from build123d import *

# Parameters (mm, degrees)
SKETCH_W        = 98
SKETCH_H        = 58
SKETCH_W_2      = 95
SKETCH_H_2      = 55
PAD_DEPTH       = 65
SKETCH001_W     = 98
SKETCH001_H     = 58
PAD001_DEPTH    = 1.5
SKETCH002_R     = 15.5
POCKET_DEPTH    = 5
SKETCH004_R     = 18.25
POCKET002_DEPTH = 0.75
SKETCH003_W     = 14.5
SKETCH003_H     = 12
SKETCH003_W_2   = 13
SKETCH003_H_2   = 6
SKETCH003_W_3   = 8
SKETCH003_H_3   = 4
POCKET003_DEPTH = 5
PAD002_DEPTH    = 3
PAD003_DEPTH    = 1


with BuildPart() as part:
    # Sketch → Pad (new body)
    with BuildSketch(Plane.XY):
        with Locations((0, -29)):
            Rectangle(SKETCH_W, SKETCH_H)
        with Locations((0, -29)):
            Rectangle(SKETCH_W_2, SKETCH_H_2, mode=Mode.SUBTRACT)
    extrude(amount=PAD_DEPTH)

    # Sketch001 → Pad001 (join)
    with BuildSketch(Plane.XY):
        with Locations((0, -29)):
            Rectangle(SKETCH001_W, SKETCH001_H)
    extrude(amount=PAD001_DEPTH)

    # Sketch002 → Pocket (cut)
    with BuildSketch(Plane.XZ):
        with Locations((0, 30)):
            Circle(SKETCH002_R)
    extrude(amount=POCKET_DEPTH, mode=Mode.SUBTRACT)

    # Sketch004 → Pocket002 (cut)
    with BuildSketch(Plane.XZ.offset(1.5)):
        with Locations((0, 30)):
            Circle(SKETCH004_R)
    extrude(amount=-POCKET002_DEPTH, mode=Mode.SUBTRACT)

    # Sketch003 → Pocket003 (cut)
    with BuildSketch(Plane.XY):
        with Locations((0, -8.5)):
            Rectangle(SKETCH003_W, SKETCH003_H)
        with Locations((31, -46)):
            Rectangle(SKETCH003_W_2, SKETCH003_H_2)
        with Locations((16.2, -46)):
            Rectangle(SKETCH003_W_3, SKETCH003_H_3)
    extrude(amount=POCKET003_DEPTH, mode=Mode.SUBTRACT)

    # Sketch005 → Pad002 (join)
    with BuildSketch(Plane.XZ):
        with BuildLine():
            ThreePointArc((23.5, 30), (0, 53.5), (-23.5, 30))
            Line((-25, 30), (-23.5, 30))
            ThreePointArc((25, 30), (0, 55), (-25, 30))
            Line((23.5, 30), (25, 30))
        make_face()
    extrude(amount=-PAD002_DEPTH)

    # Sketch006 (on Face33 of Pad002) → Pad003 (join)
    with BuildSketch(Plane(origin=(0, 3, 0), x_dir=(-1, 0, 0), z_dir=(0, 1, 0))):
        with BuildLine():
            ThreePointArc((26.5, 30), (0, 56.5), (-26.5, 30))
            Line((-26.5, 30), (-23.5, 30))
            ThreePointArc((23.5, 30), (0, 53.5), (-23.5, 30))
            Line((23.5, 30), (26.5, 30))
        make_face()
    extrude(amount=-PAD003_DEPTH)


solid = part.part
Read the model definition and answer for the solid it produces. Units are mm, in the model's axes. A direction names the side the tool comes from. Round coordinates to 2 decimals unless told otherwise and drop trailing zeros. Write each loop counter-clockwise with the first axis right and the second up, starting at its lowest first coordinate (ties: lowest second). Pieces come first, ordered by that corner, then holes. Notation, with made-up numbers: (1, 16.25) - (10, 16.25) arc R26 ccw to (10, 55.25) - close; hole circle Ø8 at (4.5, -7.5). An arc over 180 degrees is marked (long way). One line per question, with ' | ' between items. Start each with the question number.
1. Section B-B (z = 6.5) is taken. Determine the outline of the cut face in (x, y).
2. Section C-C (y = -10) is taken. Determine the outline of the cut face in (x, z), and give its area (3 significant figures).
3. Find the intervals of material crossed by probe 1 along Y at (x, z) = (-23.5, 10); probe 2 along X at (y, z) = (-5.5, 17.5); probe 3 along Y at (x, z) = (-14.5, 24), in increasing order. Write a range as [from, to].
4. Section A-A (x = 0) is taken. Determine the outline of the cut face in (y, z).
5. Section D-D (x = -10) is taken. Determine the outline of the cut face in (y, z).
6. This flat-tipped pin is pushed along its axis until it touches: pin 1 (1.5 mm diameter, centred on x = -35.5, y = -7, fed in from +Z). Where does it stop, or does it pass through?
7. For faces 1 (the face through (24.7, 1.9, 30)), 2 (the face through (-11, -1.5, 47)), 3 (the face through (-3.956, -1.13, 12.184)), 4 (the face through (0.517, 1.479, 53.494)), 5 (the face through (-0.583, 2.507, 56.494)), determine the directions among +Z, -Z, +X, -X, +Y, -Y from which every point of the face is accessible in a straight line to the end or side of a thin tool.
8. For a pull along Z with two mould halves and no side action, classify faces 6 (the face through (0.55, 0.986, 54.994)), 7 (the face through (-8.2, -0.75, 16.6)), 8 (the face through (-24.6, 1.9, 30)) as +Z half, -Z half, draft (parallel to the pull), parting line (faces both ways), or undercut.
Filled in:
1) outline: (-49, -58) - (49, -58) - (49, 0) - (-49, 0) - close; hole (-47.5, -56.5) - (47.5, -56.5) - (47.5, -1.5) - (-47.5, -1.5) - close
2) outline: (-49, 0) - (-7.25, 0) - (-7.25, 1.5) - (-47.5, 1.5) - (-47.5, 65) - (-49, 65) - close; (7.25, 0) - (49, 0) - (49, 65) - (47.5, 65) - (47.5, 1.5) - (7.25, 1.5) - close | area: 316 mm²
3) probe 1: [-58, -56.5], [-1.5, 0] | probe 2: [-49, -47.5], [47.5, 49] | probe 3: [-58, -56.5], [-0.75, 0]
4) outline: (-58, 0) - (-14.5, 0) - (-14.5, 1.5) - (-56.5, 1.5) - (-56.5, 65) - (-58, 65) - close; (-2.5, 0) - (0, 0) - (0, 14.5) - (-0.75, 14.5) - (-0.75, 11.75) - (-1.5, 11.75) - (-1.5, 1.5) - (-2.5, 1.5) - close; (-1.5, 48.25) - (-0.75, 48.25) - (-0.75, 45.5) - (0, 45.5) - (0, 53.5) - (3, 53.5) - (3, 56.5) - (2, 56.5) - (2, 55) - (0, 55) - (0, 65) - (-1.5, 65) - close
5) outline: (-58, 0) - (0, 0) - (0, 18.16) - (-0.75, 18.16) - (-0.75, 14.73) - (-1.5, 14.73) - (-1.5, 1.5) - (-56.5, 1.5) - (-56.5, 65) - (-58, 65) - close; (-1.5, 45.27) - (-0.75, 45.27) - (-0.75, 41.84) - (0, 41.84) - (0, 51.27) - (3, 51.27) - (3, 54.54) - (2, 54.54) - (2, 52.91) - (0, 52.91) - (0, 65) - (-1.5, 65) - close
6) pin 1: z = 1.5
7) face 1: -Z, +X, -X, +Y | face 2: +Z | face 3: none | face 4: -Z, +Y | face 5: +Z, +Y
8) face 6: +Z half | face 7: undercut | face 8: -Z half
